```python
from build123d import *

# Parameters (mm, degrees)
F0_W = 4.3428323324
F0_H = 0.9698241177
F2_R = 2


with BuildPart() as f1:
    # F0 (on Front) → F1 (revolve)
    with BuildSketch(Plane.XZ):
        Polygon((0, 41.463367641), (-2.7215683367, 41.463367641), (-3.2072065232, 41.463367641), (-3.2072065232, 35.3673755124), (-4.7536900101, 31.317062021), (-4.7536900101, 4.4173045305), (-4.3428323324, 4.4173045305), (0, 4.4173045305), align=None)
        with Locations((-2.1714161662, 3.9323924717)):
            Rectangle(F0_W, F0_H)
        Polygon((0, 2.1724704409), (0, 3.4474804128), (-4.3428323324, 3.4474804128), (-4.7536900101, 3.4474804128), (-4.7536900101, 2.1724704409), align=None)
    revolve(axis=Axis((0, 0, 29.95), (0, 0, 1)))

    # F2
    f2_edges = [f1.edges().sort_by_distance(p)[0] for p in [
        (3.207207, 0, 35.367376),
        (4.75369, 0, 31.317062),
    ]]
    fillet(f2_edges, radius=F2_R)

    # F0 (on Front) → F3 (revolve)
    with BuildSketch(Plane.XZ):
        with BuildLine():
            Line((0, 41.463367641), (0, 58.5273988545))
            add(Edge.make_bspline(
                [(0, 58.5273988545), (-0.36253144, 58.486839259), (-1.1596346327, 58.3977811986), (-1.1249576474, 56.6070187801), (-2.3576224657, 52.9317939751), (-2.579834999, 45.9332704529), (-2.7215683367, 41.463367641)],
                knots=[0, 0, 0, 0, 0.1308182588, 0.2872358796, 0.5423006179, 1, 1, 1, 1], degree=3))
            Line((-2.7215683367, 41.463367641), (0, 41.463367641))
        make_face()
    revolve(axis=Axis((0, 0, 29.95), (0, 0, 1)))


solid = f1.part
```
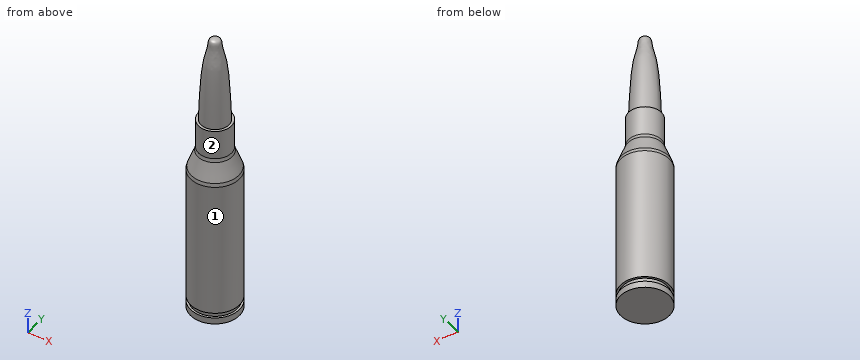
Geometry check sheet. Reference: the model listing, model coordinates, mm. Face numbers are marked on the shaded views. A direction names the side the tool comes from. Round coordinates to 2 decimals unless told otherwise and drop trailing zeros. Loops run counter-clockwise (first coordinate to the right, second up) from the corner with the lowest first, then second, coordinate; pieces in that order, holes last. Notation, with made-up numbers: (-17.5, 37.5) -> (-9.5, 37.5) arc R20 ccw to (-9.5, 56.5) -> close; hole circle Ø1 at (44.5, 58). An arc over 180 degrees is marked (long way). Use a Markdown table: item, result.
(1) Go/stop test with flat-tipped pins: P1, Ø4, axis at y = -3.5, z = 52, coming from the -X side; P2, Ø5, axis at x = -1.5, z = 24.5, coming from the -Y side; P3, Ø4, axis at x = 3.5, z = 19, coming from the +Y side. Record where each tip stops, or that it passes through.
Calculated:
| item | result |
|---|---|
| P1 | x = -1.56 |
| P2 | y = -4.75 |
| P3 | y = 4.51 |
(2) Scan lines: probe 1 along Z at (x, y) = (-1, 3); probe 2 along Z at (x, y) = (3, -3.25); probe 3 along Y at (x, z) = (2.75, 13). Record each from-to range of solid material in increasing order.
Calculated:
| item | result |
|---|---|
| probe 1 | 2.17 to 41.46 |
| probe 2 | 2.17 to 3.45, 4.42 to 32.18 |
| probe 3 | -3.88 to 3.88 |
(3) Sectioned sample at A-A (z = 14). Enter the section's corners in (x, y), then the cut area to 3 significant figures.
Calculated:
| item | result |
|---|---|
| outline | circle Ø9.51 at (0, 0) |
| area | 71.0 mm² |
(4) Set-up check for the marked faces 1 and 2: record each of +Z, -Z, +X, -X, +Y, -Y from which the full face is reachable in a straight line by a thin tool's end or side.
Calculated:
| item | result |
|---|---|
| face 1 | +Z, -Z |
| face 2 | +Z |
(5) Sectioned sample at B-B (z = 33). Enter the section's corners in (x, y), then the cut area to 3 significant figures.
Calculated:
| item | result |
|---|---|
| outline | circle Ø8.22 at (0, 0) |
| area | 53.1 mm² |
